Here's how the part is built. I have some questions about the finished solid (model axes, mm). Give positions to 0.01 mm unless a question says otherwise; leave off trailing zeros. Loops run counter-clockwise (first coordinate to the right, second up) from the corner with the lowest first, then second, coordinate; pieces in that order, holes last. Notation, with made-up numbers: (82.5, 37.5) - (91.5, 37.5) arc R15 ccw to (91.5, 54.5) - close; hole circle Ø6 at (77, 62.25). An arc over 180 degrees is marked (long way). Use one line per item in the form item = value.
from build123d import *

# Parameters (mm, degrees)
SKETCH1_W           = 50.8
SKETCH1_H           = 50.8
SKETCH1_W_2         = 47.625
SKETCH1_H_2         = 47.625
BOSS_EXTRUDE1_DEPTH = 101.6
SKETCH2_R           = 2.54
CUT_EXTRUDE2_DEPTH  = 609.6


with BuildPart() as part:
    # Sketch1 → Boss-Extrude1 (new body)
    with BuildSketch(Plane(origin=(0, 0, 0), x_dir=(0, 0, -1), z_dir=(1, 0, 0))):
        Rectangle(SKETCH1_W, SKETCH1_H)
        Rectangle(SKETCH1_W_2, SKETCH1_H_2, mode=Mode.SUBTRACT)
    extrude(amount=BOSS_EXTRUDE1_DEPTH)

    # Sketch2 → Cut-Extrude2 (cut)
    with BuildSketch(Plane.XY.offset(25.4)):
        with Locations((12.7, 12.7)):
            Circle(SKETCH2_R)
        with Locations((12.7, 0)):
            Circle(SKETCH2_R)
        with Locations((12.7, -12.7)):
            Circle(SKETCH2_R)
        with Locations((25.4, 12.7)):
            Circle(SKETCH2_R)
        with Locations((25.4, 0)):
            Circle(SKETCH2_R)
        with Locations((25.4, -12.7)):
            Circle(SKETCH2_R)
        with Locations((38.1, 12.7)):
            Circle(SKETCH2_R)
        with Locations((38.1, 0)):
            Circle(SKETCH2_R)
        with Locations((38.1, -12.7)):
            Circle(SKETCH2_R)
        with Locations((50.8, 12.7)):
            Circle(SKETCH2_R)
        with Locations((50.8, 0)):
            Circle(SKETCH2_R)
        with Locations((50.8, -12.7)):
            Circle(SKETCH2_R)
        with Locations((63.5, 12.7)):
            Circle(SKETCH2_R)
        with Locations((63.5, 0)):
            Circle(SKETCH2_R)
        with Locations((63.5, -12.7)):
            Circle(SKETCH2_R)
        with Locations((76.2, 12.7)):
            Circle(SKETCH2_R)
        with Locations((76.2, 0)):
            Circle(SKETCH2_R)
        with Locations((76.2, -12.7)):
            Circle(SKETCH2_R)
        with Locations((88.9, 12.7)):
            Circle(SKETCH2_R)
        with Locations((88.9, 0)):
            Circle(SKETCH2_R)
        with Locations((88.9, -12.7)):
            Circle(SKETCH2_R)
    extrude(amount=-CUT_EXTRUDE2_DEPTH, mode=Mode.SUBTRACT)


solid = part.part
(1) If we section it at A-A (z = 18): List the corners of the cut face in (x, y) for me, plus the area to 3 significant figures.
Geometry says:
outline = (0, -25.4) - (101.6, -25.4) - (101.6, -23.81) - (0, -23.81) - close; (0, 23.81) - (101.6, 23.81) - (101.6, 25.4) - (0, 25.4) - close
area = 323 mm²
(2) If we section it at C-C (x = 25.4): Give the number of separate pieces and of enclosed holes in the cut face, plus the area to 3 significant figures.
Geometry says:
separate_pieces = 6
enclosed_holes = 0
area = 264 mm²
(3) If I drill on probe 1 along Y at (x, z) = (88.9, -24.65); probe 2 along Y at (x, z) = (26, -9), over which ranges is the centre line in solid material (lowest first)?
Geometry says:
probe_1 = -25.4 to -15.24, -10.16 to -2.54, 2.54 to 10.16, 15.24 to 25.4
probe_2 = -25.4 to -23.81, 23.81 to 25.4
(4) Thinking about a two-plate mould opening in Y: for faces 1 (the flat face through (50, 5, -25.4)), 2 (the flat face through (50, 25.4, 0)), 3 (the cylindrical face through (10.684, -1.546, 24.617)), which applies, pulls with the +Y half, pulls with the -Y half, needs draft (parallel to the pull), parting line crosses it, or undercut?
Geometry says:
face_1 = needs draft
face_2 = pulls with the +Y half
face_3 = undercut
